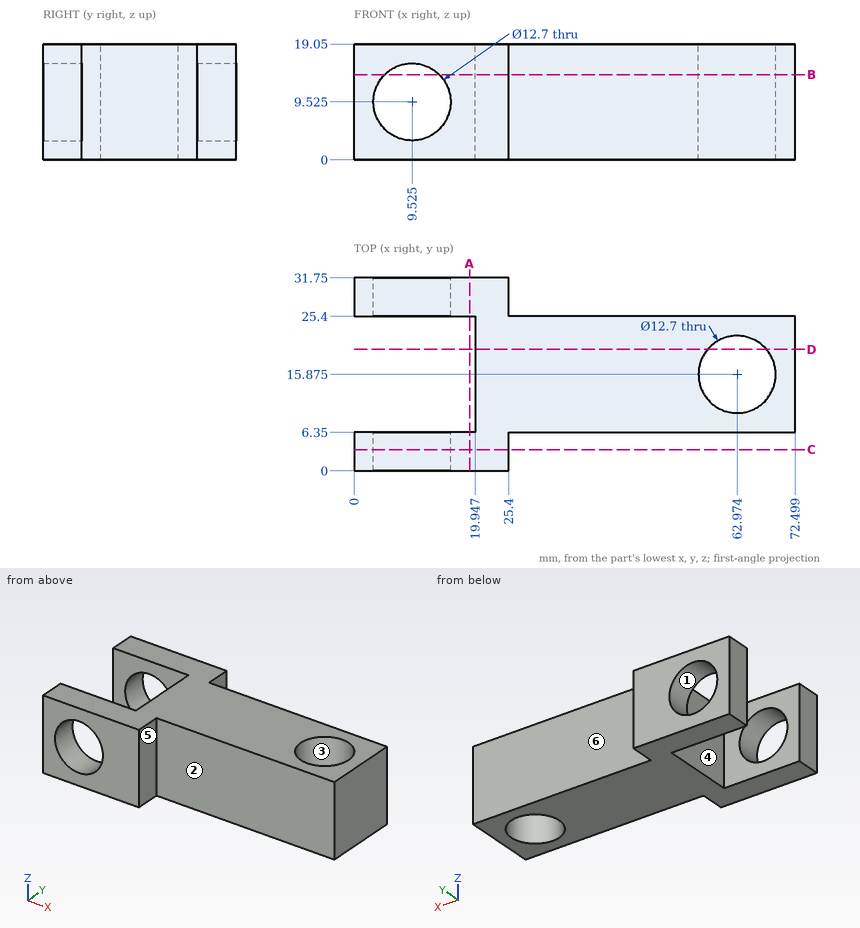
Geometry: see drawing. Coordinates: mm, zero at the bounding-box minimum. A direction names the side the tool comes from. Give positions to 0.01 mm unless a question says otherwise; leave off trailing zeros. Order: outer loops, then holes, each group sorted by start corner. A loop starts at its lowest first (then second) coordinate and runs counter-clockwise, first axis right, second up.
Q1. Set-up query: the marked faces 4, 5 and 6. Return all of +Z, -Z, +X, -X, +Y, -Y with unobstructed straight access to the full face (end or side cutting, diameter ignored); none if empty.
Checked values:
face 4: +Z, -Z, -X
face 5: +Z, -Z, +X, -Y
face 6: +Z, -Z, +X, +Y
Q2. Section B-B on z = 14. State how many separate pieces and enclosed holes the cut face has, and give its area (3 significant figures).
Checked values:
separate pieces: 3
enclosed holes: 1
area: 1,080 mm2
Q3. Ray query, probe 1 along X at (y, z) = (23, 14.5); probe 2 along Y at (x, z) = (55, 17.75); probe 3 along X at (y, z) = (29.5, 10.25). Return the intervals inside material, ascending.
Checked values:
probe 1: x = 19.95 to 72.5
probe 2: y = 6.35 to 25.4
probe 3: x = 0 to 3.22, 15.83 to 25.4
Q4. Section D-D on y = 20. Output: boundary loops of the cut face in (x, z).
Checked values:
outline: (19.95, 0) - (58.15, 0) - (58.15, 19.05) - (19.95, 19.05) - close; (67.8, 0) - (72.5, 0) - (72.5, 19.05) - (67.8, 19.05) - close
Q5. Draft query along Y for the marked faces 1, 2 and 3. Return one class per face: +Y half, -Y half, draft (parallel to the pull), parting line (faces both ways), or undercut.
Checked values:
face 1: draft
face 2: -Y half
face 3: undercut
Q6. Contact query for flat-ended pins moving along their axis: pin 1 Ø9.5 at (x, z) = (42.5, 9.5) entering from -Y; pin 2 Ø2 at (y, z) = (28, 14) entering from +X. Output: stop coordinate, or through.
Checked values:
pin 1: stops at y = 6.35
pin 2: stops at x = 25.4
Q7. Section A-A on x = 19. Output: boundary loops of the cut face in (y, z).
Checked values:
outline: (0, 0) - (6.35, 0) - (6.35, 19.05) - (0, 19.05) - close; (25.4, 0) - (31.75, 0) - (31.75, 19.05) - (25.4, 19.05) - close
Q8. Section C-C on y = 3.5. Output: boundary loops of the cut face in (x, z) (3 decimals).
Checked values:
outline: (0, 0) - (25.4, 0) - (25.4, 19.05) - (0, 19.05) - close; hole circle Ø12.7 at (9.525, 9.525)
